```python
from build123d import *

# Parameters (mm, degrees)
SKETCH1_R             = 5
BOSS_EXTRUDE1_DEPTH   = 200
SKETCH2_R             = 7.5
BOSS_EXTRUDE2_DEPTH   = 20
BOSS_EXTRUDE2_2_DEPTH = 20
SKETCH3_R             = 7.5
BOSS_EXTRUDE3_DEPTH   = 27.5
BOSS_EXTRUDE4_START   = 27.5
SKETCH4_R             = 7.5
BOSS_EXTRUDE4_DEPTH   = 27.5
SKETCH5_R             = 5
CUT_EXTRUDE1_DEPTH    = 239.497903555


with BuildPart() as part:
    # Sketch1 → Boss-Extrude1 (new, symmetric)
    with BuildSketch(Plane(origin=(0, 0, 0), x_dir=(0, 0, -1), z_dir=(1, 0, 0))):
        Circle(SKETCH1_R)
    extrude(amount=BOSS_EXTRUDE1_DEPTH, both=True)



with BuildPart() as body_2:
    # Sketch2 → Boss-Extrude2 (new, symmetric)
    with BuildSketch(Plane(origin=(0, 0, 0), x_dir=(1, 0, 0), z_dir=(0, 1, 0))):
        with Locations(Location((227.5, 0, 0), (0, 0, 270))):
            Circle(SKETCH2_R)
    extrude(amount=BOSS_EXTRUDE2_DEPTH, both=True)


with BuildPart() as body_3:
    # Sketch2 → Boss-Extrude2 2 (new, symmetric)
    with BuildSketch(Plane(origin=(0, 0, 0), x_dir=(1, 0, 0), z_dir=(0, 1, 0))):
        with Locations(Location((-227.5, 0, 0), (0, 0, 90))):
            Circle(SKETCH2_R)
    extrude(amount=BOSS_EXTRUDE2_2_DEPTH, both=True)


with BuildPart() as part_1:
    add(part.part)

    add(body_3.part)  # Boss-Extrude3 merges body 3
    # Sketch3 → Boss-Extrude3 (add)
    with BuildSketch(Plane.ZY.offset(200)):
        Circle(SKETCH3_R)
    extrude(amount=BOSS_EXTRUDE3_DEPTH)


    add(body_2.part)  # Boss-Extrude4 merges body 2
    # Sketch4 → Boss-Extrude4 (add)
    with BuildSketch(Plane(origin=(200, 0, 0), x_dir=(0, 0, -1), z_dir=(1, 0, 0)).offset(BOSS_EXTRUDE4_START)):
        Circle(SKETCH4_R)
    extrude(amount=-BOSS_EXTRUDE4_DEPTH)

    # Sketch5 → Cut-Extrude1 (cut, through all)
    with BuildSketch(Plane(origin=(0, 20, 0), x_dir=(1, 0, 0), z_dir=(0, 1, 0))):
        with Locations(Location((227.5, 0, 0), (0, 0, 270))):
            Circle(SKETCH5_R)
        with Locations(Location((-227.5, 0, 0), (0, 0, 90))):
            Circle(SKETCH5_R)
    extrude(amount=-CUT_EXTRUDE1_DEPTH, mode=Mode.SUBTRACT)


solid = part_1.part
```
Geometry check sheet. Reference: the model listing, model coordinates, mm. A direction names the side the tool comes from. Give positions to 0.01 mm unless a question says otherwise; leave off trailing zeros. Loops run counter-clockwise (first coordinate to the right, second up) from the corner with the lowest first, then second, coordinate; pieces in that order, holes last. Notation, with made-up numbers: M 22,7.25 L 51,7.25 A26 ccw 51,32.25 Z; hole C 5.25,20 d6. An arc over 180 degrees is marked long. Answer as CSV lines item,"result".
Item 1: Cross-section at A-A on z = 0. Record the cut outline in (x, y), and give its area (3 significant figures).
Values:
outline,"M -235,-20 L -232.5,-20 L -232.5,20 L -235,20 Z; M -222.5,-20 L -220,-20 L -220,-7.5 L -200,-7.5 L -200,-5 L 200,-5 L 200,-7.5 L 220,-7.5 L 220,-20 L 222.5,-20 L 222.5,20 L 220,20 L 220,7.5 L 200,7.5 L 200,5 L -200,5 L -200,7.5 L -220,7.5 L -220,20 L -222.5,20 Z; M 232.5,-20 L 235,-20 L 235,20 L 232.5,20 Z"
area,"5,000 mm²"
Item 2: Release check for a two-part mould opening along X. For faces 3 (the cylindrical face through (232.457, 0.28, -0.651)), 4 (the flat face through (222.6, -20, 1.6)) record: pulls with the +X half, pulls with the -X half, needs draft (parallel to the pull), parting line crosses it, or undercut.
Values:
face 3,"undercut"
face 4,"needs draft"
Item 3: Cross-section at B-B on y = 0. Record the cut outline in (x, z).
Values:
outline,"M -227.5,-7.5 L -200,-7.5 L -200,-5 L 200,-5 L 200,-7.5 L 227.5,-7.5 A7.5 ccw 227.5,7.5 L 200,7.5 L 200,5 L -200,5 L -200,7.5 L -227.5,7.5 A7.5 ccw Z; hole C -227.5,0 d10; hole C 227.5,0 d10"
Item 4: Material ranges on line 1 (X direction, y = -8.5, z = 0); line 2 (Z direction, x = -227.5, y = 8.5); line 3 (X direction, y = 4, z = 0), recorded low to high.
Values:
line 1,"x = -235 to -232.5, -222.5 to -220, 220 to 222.5, 232.5 to 235"
line 2,"z = -7.5 to -5, 5 to 7.5"
line 3,"x = -235 to -232.5, -222.5 to 222.5, 232.5 to 235"
Item 5: Access from +Z, -Z, +X, -X, +Y, -Y to the whole of each face (thin tool, end or side, straight path). Record for faces 1 (the flat face through (222.6, 20, 1.6)), 2 (the cylindrical face through (-210.502, -4.564, -5.952)).
Values:
face 1,"+Z, -Z, +X, -X, +Y"
face 2,"none"
Item 6: Depth check by flat-ended pin: P1, Ø5, axis at x = -9, z = 0.5, coming from the +Y side; P2, Ø4, axis at y = -11.5, z = 5, coming from the +X side; P3, Ø5, axis at x = -39.5, y = -2.5, coming from the +Z side. Enter the tip coordinate at first touch or a pass-through.
Values:
P1,"stops at y = 5"
P2,"stops at x = 234.37"
P3,"stops at z = 5"
